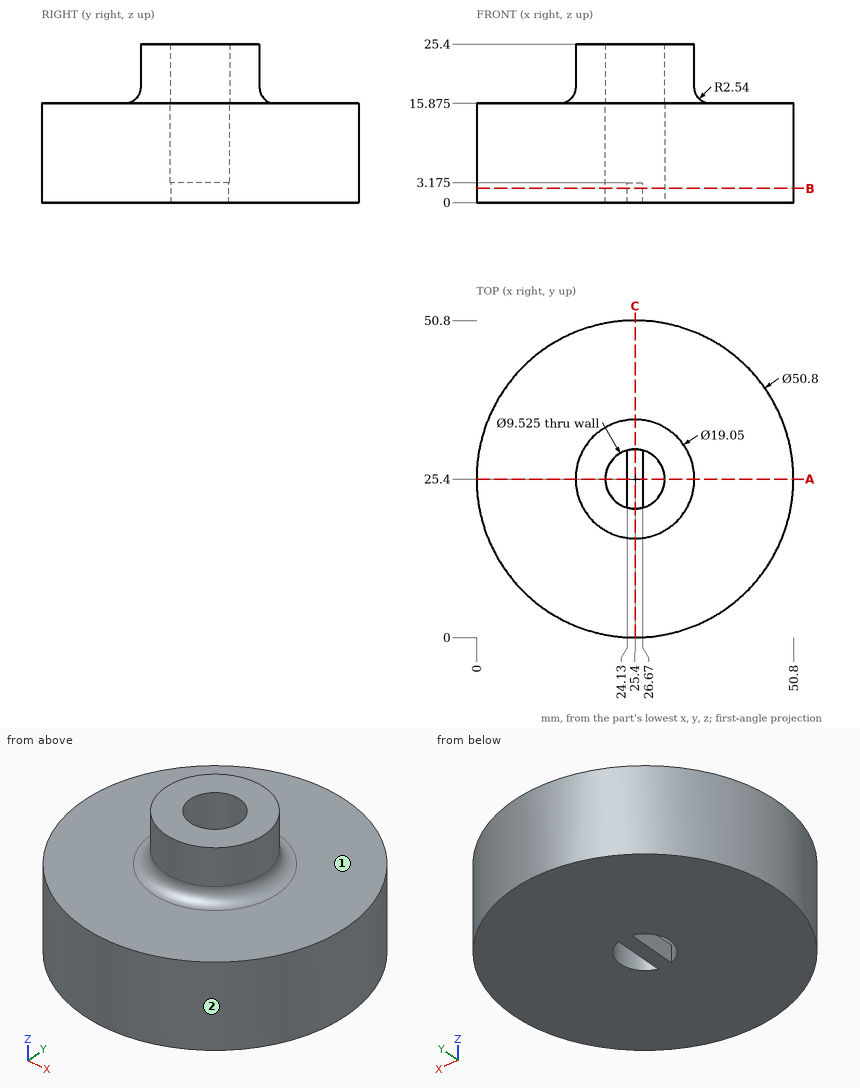
Verification items for this drawing (mm, ordinates from the low corner). A direction names the side the tool comes from. Coordinates: 2 decimals unless noted, no trailing zeros. Loops run counter-clockwise (first coordinate to the right, second up) from the corner with the lowest first, then second, coordinate; pieces in that order, holes last.
Item 1: Sectioned sample at B-B, the plane z = 2.25. Record the boundary of the cut face in (x, y) (1 decimal), then the cut area to 3 significant figures.
Item 2: Access from +Z, -Z, +X, -X, +Y, -Y to the whole of each face (thin tool, end or side, straight path). Record for the marked faces 1 and 2.
Item 3: Thickness scan on line 1 (Y direction, x = 25.4, z = 6.5); line 2 (Z direction, x = 48, y = 25) (3 decimals). Record the ranges inside material, lowest first.
Item 4: Sectioned sample at A-A, the plane y = 25.4. Record the boundary of the cut face in (x, z) (1 decimal), then the cut area to 3 significant figures.
Item 5: Go/stop test with flat-tipped pins: pin 1 Ø1 at (x, z) = (37.5, 12.5) entering from +Y; pin 2 Ø1.6 at (y, z) = (23, 1.5) entering from -X; pin 3 Ø15 at (x, y) = (25.4, 25.4) entering from +Z; pin 4 Ø1.3 at (x, y) = (25.5, 25.5) entering from +Z (3 decimals). Record where each tip stops, or that it passes through.
Item 6: Sectioned sample at C-C, the plane x = 25.4. Record the boundary of the cut face in (y, z) (1 decimal), then the cut area to 3 significant figures.
Check result:
1. outline: circle Ø50.8 at (25.4, 25.4); hole (24.1, 20.8) - (24.1, 30) arc R4.8 ccw to start; hole (26.7, 20.8) arc R4.8 ccw to (26.7, 30) - close
1. area: 1,980 mm2
2. face 1: +Z
2. face 2: +Z, -Z
3. line 1: y = 0 to 20.64, 30.16 to 50.8
3. line 2: z = 0 to 15.875
4. outline: (0, 0) - (20.6, 0) - (20.6, 25.4) - (15.9, 25.4) - (15.9, 18.4) arc R2.5 cw to (13.3, 15.9) - (0, 15.9) - close; (24.1, 0) - (26.7, 0) - (26.7, 3.2) - (24.1, 3.2) - close; (30.2, 0) - (50.8, 0) - (50.8, 15.9) - (37.5, 15.9) arc R2.5 cw to (34.9, 18.4) - (34.9, 25.4) - (30.2, 25.4) - close
4. area: 757 mm2
5. pin 1: stops at y = 48
5. pin 2: stops at x = 0.05
5. pin 3: stops at z = 25.4
5. pin 4: stops at z = 3.175
6. outline: (0, 0) - (50.8, 0) - (50.8, 15.9) - (37.5, 15.9) arc R2.5 cw to (34.9, 18.4) - (34.9, 25.4) - (30.2, 25.4) - (30.2, 3.2) - (20.6, 3.2) - (20.6, 25.4) - (15.9, 25.4) - (15.9, 18.4) arc R2.5 cw to (13.3, 15.9) - (0, 15.9) - close
6. area: 779 mm2
